CAD build for the part. Positions are in the model's coordinates, mm. A direction names the side the tool comes from. Coordinates: 2 decimals unless noted, no trailing zeros. Order: outer loops, then holes, each group sorted by start corner. A loop starts at its lowest first (then second) coordinate and runs counter-clockwise, first axis right, second up. Notation, with made-up numbers: (-0.5, 42.25) - (58.5, 42.25) arc R34 ccw to (58.5, 74.25) - close; hole circle Ø4 at (39, 5). An arc over 180 degrees is marked (long way). Return JSON: item names as keys, results as strings.
from build123d import *

# Parameters (mm, degrees)
SKETCH1_W           = 44.45
SKETCH1_H           = 50.8
BOSS_EXTRUDE1_DEPTH = 76.2
CUT_EXTRUDE1_REACH  = 93.801
SKETCH2_R           = 6.731
SKETCH3_R           = 9.906
CUT_EXTRUDE2_DEPTH  = 38.608
CUT_EXTRUDE3_DEPTH  = 6.35
SKETCH5_R           = 12.0142
CUT_EXTRUDE4_DEPTH  = 3.81
SKETCH6_R           = 14.6812
CUT_EXTRUDE5_DEPTH  = 1.5875


with BuildPart() as part:
    # Sketch1 → Boss-Extrude1 (new, symmetric)
    with BuildSketch(Plane.XY):
        Rectangle(SKETCH1_W, SKETCH1_H)
    extrude(amount=BOSS_EXTRUDE1_DEPTH, both=True)

    # Sketch2 → Cut-Extrude1 (cut, up to next)
    with BuildSketch(Plane(origin=(22.225, 0, 0), x_dir=(0, 0, -1), z_dir=(1, 0, 0)), mode=Mode.PRIVATE) as cut_extrude1_sk1:
        with Locations((-49.2125, -1.524)):
            Circle(SKETCH2_R)
    cut_extrude1_tool1 = extrude(cut_extrude1_sk1.sketch, amount=-CUT_EXTRUDE1_REACH, mode=Mode.PRIVATE) & part.part
    # Sketch2 → Cut-Extrude1 (cut, up to next)
    with BuildSketch(Plane(origin=(22.225, 0, 0), x_dir=(0, 0, -1), z_dir=(1, 0, 0)), mode=Mode.PRIVATE) as cut_extrude1_sk2:
        with Locations((49.2125, -1.524)):
            Circle(SKETCH2_R)
    cut_extrude1_tool2 = extrude(cut_extrude1_sk2.sketch, amount=-CUT_EXTRUDE1_REACH, mode=Mode.PRIVATE) & part.part
    add(cut_extrude1_tool1.solids().sort_by_distance((22.225, -1.524, 49.2125))[0], mode=Mode.SUBTRACT)
    add(cut_extrude1_tool2.solids().sort_by_distance((22.225, -1.524, -49.2125))[0], mode=Mode.SUBTRACT)

    # Sketch3 → Cut-Extrude2 (cut)
    with BuildSketch(Plane(origin=(22.225, 0, 0), x_dir=(0, 0, -1), z_dir=(1, 0, 0))):
        with Locations((-49.2125, -1.524)):
            Circle(SKETCH3_R)
        with Locations((49.2125, -1.524)):
            Circle(SKETCH3_R)
    extrude(amount=-CUT_EXTRUDE2_DEPTH, mode=Mode.SUBTRACT)

    # Sketch4 → Cut-Extrude3 (cut)
    with BuildSketch(Plane.XZ.offset(25.4)):
        with BuildLine():
            Line((22.225, -12.890241244), (22.225, 21.531765175))
            Line((22.225, 21.531765175), (0.947246364, 18.89010908))
            ThreePointArc((0.947246364, 18.89010908), (-11.925153457, 4.320761965), (0.947246364, -10.248585149))
            Line((0.947246364, -10.248585149), (22.225, -12.890241244))
        make_face()
    extrude(amount=-CUT_EXTRUDE3_DEPTH, mode=Mode.SUBTRACT)

    # Sketch5 → Cut-Extrude4 (cut)
    with BuildSketch(Plane.XZ.offset(19.05)):
        with Locations((2.756046543, 4.320761965)):
            Circle(SKETCH5_R)
    extrude(amount=-CUT_EXTRUDE4_DEPTH, mode=Mode.SUBTRACT)

    # Sketch6 → Cut-Extrude5 (cut)
    with BuildSketch(Plane.XZ.offset(19.05)):
        with Locations((2.756046543, 4.320761965)):
            Circle(SKETCH6_R)
    extrude(amount=-CUT_EXTRUDE5_DEPTH, mode=Mode.SUBTRACT)


solid = part.part
Item 1: Drop flat-ended pins along their axis: P1, Ø12, axis at y = -1.52, z = -49.21, coming from the -X side; P2, Ø15.5, axis at y = -1.52, z = 49.21, coming from the +X side; P3, Ø14.5, axis at x = 1.5, z = 10, coming from the -Y side. Give the stop position or say it passes through.
Findings below:
{"P1": "passes through", "P2": "stops at x = -16.38", "P3": "stops at y = -17.46"}
Item 2: Wall check: L1, parallel to Z at x = 8, y = -6.5; L2, parallel to Z at x = 6.5, y = -8.5; L3, parallel to Y at x = -1.5, z = -4.5. Give the ranges that are in metal, low to high. Write a range as [from, to].
Findings below:
{"L1": "z = [-76.2, -57.78], [-40.65, 40.65], [57.78, 76.2]", "L2": "z = [-76.2, -56.25], [-42.18, 42.18], [56.25, 76.2]", "L3": "y = [-15.24, 25.4]"}
Item 3: Band-saw the part on D-D, the plane z = -50. List the corners of the cut face in (x, y) (3 decimals), then the cut area to 3 significant figures.
Findings below:
{"outline": "(-22.225, -25.4) - (22.225, -25.4) - (22.225, -11.399) - (-16.383, -11.399) - (-16.383, -8.209) - (-22.225, -8.209) - close; (-22.225, 5.161) - (-16.383, 5.161) - (-16.383, 8.351) - (22.225, 8.351) - (22.225, 25.4) - (-22.225, 25.4) - close", "area": "1,420 mm²"}
Item 4: Band-saw the part on A-A, the plane y = -22. List the corners of the cut face in (x, z) (3 decimals).
Findings below:
{"outline": "(-22.225, -76.2) - (22.225, -76.2) - (22.225, -12.89) - (0.947, -10.249) arc R14.681 cw to (0.947, 18.89) - (22.225, 21.532) - (22.225, 76.2) - (-22.225, 76.2) - close"}
Item 5: Mould opens along Y. For faces 4 (the flat face through (0, 25.4, 1)), 5 (the flat face through (3, -15.24, 4)), 6 (the cylindrical face through (9.215, -16.367, 14.451)), 7 (the flat face through (-16.383, -8, 52)) say: released by +Y, released by -Y, zero draft, split by the parting line, or undercut.
Findings below:
{"face 4": "released by +Y", "face 5": "released by -Y", "face 6": "zero draft", "face 7": "undercut"}
Item 6: Band-saw the part on B-B, the plane x = -0.5. List the corners of the cut face in (y, z), then the cut area to 3 significant figures.
Findings below:
{"outline": "(-25.4, -76.2) - (25.4, -76.2) - (25.4, 76.2) - (-25.4, 76.2) - (-25.4, 18.64) - (-17.46, 18.64) - (-17.46, 15.89) - (-15.24, 15.89) - (-15.24, -7.24) - (-17.46, -7.24) - (-17.46, -9.99) - (-25.4, -9.99) - close; hole circle Ø19.81 at (-1.52, -49.21); hole circle Ø19.81 at (-1.52, 49.21)", "area": "6,850 mm²"}
Item 7: Which spindle directions (+Z, -Z, +X, -X, +Y, -Y) get a long thin tool onto all of the face, cutting with end or side? Do faces 1 (the cylindrical face through (3.191, -1.088, -39.316)), 2 (the flat face through (5, -17.463, -8)), 3 (the flat face through (11.74, -22.27, 20.23)). Say none if no direction does.
Findings below:
{"face 1": "+X", "face 2": "-Y", "face 3": "+X, -Y"}
